Part print with two shaded views. Sizes in mm from the minimum x, y, z corner. A direction names the side the tool comes from. Round coordinates to 2 decimals unless told otherwise and drop trailing zeros. Order: outer loops, then holes, each group sorted by start corner. A loop starts at its lowest first (then second) coordinate and runs counter-clockwise, first axis right, second up. Notation, with made-up numbers: (69, 7) -> (92, 7) arc R14 cw to (92, 28) -> close; hole circle Ø11 at (-27, 83.25). An arc over 180 degrees is marked (long way). Put each result on its own line as item: value. Start each with the question number.
Q1. Cut at C-C, the plane z = 3.4. List the corners of the cut face in (x, y) (1 decimal).
Q2. Flat gauge pins, fed straight in: P1, Ø1.7, axis at y = 12, z = 2, coming from the +X side; P2, Ø2, axis at x = 2.5, z = 3, coming from the +Y side (1 decimal); P3, Ø2.5, axis at x = 9.5, z = 9, coming from the -Y side. Where does each tip first touch, or does it go through?
Q3. Cut at D-D, the plane x = 15.5. List the corners of the cut face in (y, z).
Q4. 3-axis set-ups, long thin cutter, end or side, ignore diameter. For the marked faces 1, 2 and 3: which of +Z, -Z, +X, -X, +Y, -Y reach the whole face in a straight line?
Q5. Cut at A-A, the plane z = 1. List the corners of the cut face in (x, y) (1 decimal).
Q6. Pull direction Y, two halves, no side cores. Call the marked faces 4, 5, 6 and 7: released by +Y, released by -Y, zero draft, split by the parting line, or undercut.
Q7. Cut at B-B, the plane y = 6. List the corners of the cut face in (x, z), and give its area (3 significant figures).
Q8. Probe L1, parallel to X at y = 16.25, z = 2.5 (1 decimal); L2, parallel to X at y = 6.5, z = 6 (1 decimal); L3, parallel to Z at x = 12.25, y = 1. List the from-to ranges inside material, lowest first.
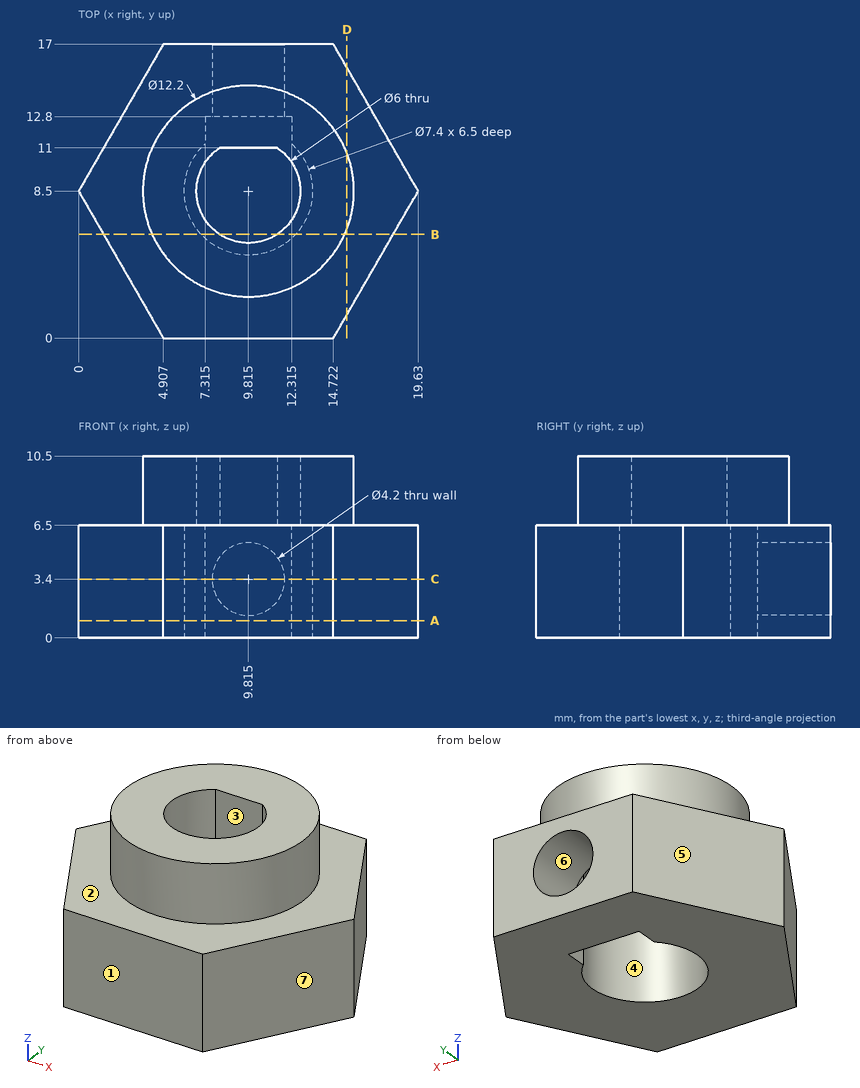
Ans:
1. outline: (0, 8.5) -> (4.9, 0) -> (14.7, 0) -> (19.6, 8.5) -> (14.7, 17) -> (11.9, 17) -> (11.9, 12.8) -> (12.3, 12.8) -> (12.3, 11.2) arc R3.7 cw (long way) to (7.3, 11.2) -> (7.3, 12.8) -> (7.7, 12.8) -> (7.7, 17) -> (4.9, 17) -> close
2. P1: stops at x = 18.1
2. P2: stops at y = 14.6
2. P3: stops at y = 2.4
3. outline: (1.35, 0) -> (15.65, 0) -> (15.65, 6.5) -> (10.71, 6.5) -> (10.71, 10.5) -> (6.29, 10.5) -> (6.29, 6.5) -> (1.35, 6.5) -> close
4. face 1: +Z, -Z, +X, -X, -Y
4. face 2: +Z
4. face 3: +Z, -Z
5. outline: (0, 8.5) -> (4.9, 0) -> (14.7, 0) -> (19.6, 8.5) -> (14.7, 17) -> (4.9, 17) -> close; hole (7.3, 11.2) arc R3.7 ccw (long way) to (12.3, 11.2) -> (12.3, 12.8) -> (7.3, 12.8) -> close
6. face 4: undercut
6. face 5: released by +Y
6. face 6: zero draft
6. face 7: released by -Y
7. outline: (1.44, 0) -> (7.09, 0) -> (7.09, 6.5) -> (8.16, 6.5) -> (8.16, 10.5) -> (4.25, 10.5) -> (4.25, 6.5) -> (1.44, 6.5) -> close; (11.47, 6.5) -> (12.54, 6.5) -> (12.54, 0) -> (18.19, 0) -> (18.19, 6.5) -> (15.38, 6.5) -> (15.38, 10.5) -> (11.47, 10.5) -> close
7. area: 105 mm^2
8. L1: x = 4.5 to 7.9, 11.7 to 15.2
8. L2: x = 1.2 to 6.7, 12.9 to 18.5
8. L3: z = 0 to 6.5
